Build history of the part. All positions in model axes, mm. A direction names the side the tool comes from. Round coordinates to 2 decimals unless told otherwise and drop trailing zeros. Write each loop counter-clockwise with the first axis right and the second up, starting at its lowest first coordinate (ties: lowest second). Pieces come first, ordered by that corner, then holes. Notation, with made-up numbers: M -6.5,-14.75 L 36.5,-14.75 A16 ccw 36.5,12.25 Z; hole C 41.25,49.25 d11. An arc over 180 degrees is marked long. One line per item, written item: value. Start each with the question number.
```python
from build123d import *

# Parameters (mm, degrees)
SKETCH1_W            = 65
SKETCH1_H            = 56
BOSS_EXTRUDE1_DEPTH  = 2
SKETCH2_R            = 1.375
CUT_EXTRUDE1_DEPTH   = 2
FILLET1_R            = 3
FILLET2_R            = 3
FILLET3_R            = 3
FILLET4_R            = 3
SKETCH3_W            = 50
SKETCH3_H            = 5
BOSS_EXTRUDE2_DEPTH  = 9
SKETCH4_W            = 3
SKETCH4_H            = 22
BOSS_EXTRUDE3_DEPTH  = 6
SKETCH5_W            = 14
SKETCH5_H            = 13
BOSS_EXTRUDE4_DEPTH  = 5
SKETCH6_W            = 6
SKETCH6_H            = 12.1
BOSS_EXTRUDE5_DEPTH  = 6
SKETCH7_R            = 2.5
BOSS_EXTRUDE6_DEPTH  = 3
SKETCH8_W            = 3
SKETCH8_H            = 22
BOSS_EXTRUDE7_DEPTH  = 6
SKETCH9_W            = 16
SKETCH9_H            = 11
BOSS_EXTRUDE8_DEPTH  = 6
SKETCH10_W           = 7
SKETCH10_H           = 6
BOSS_EXTRUDE9_DEPTH  = 3
SKETCH11_W           = 17
SKETCH11_H           = 13
BOSS_EXTRUDE10_DEPTH = 2
SKETCH12_W           = 13
SKETCH12_H           = 13
BOSS_EXTRUDE11_DEPTH = 1


with BuildPart() as part:
    # Sketch1 → Boss-Extrude1 (new body)
    with BuildSketch(Plane(origin=(0, 0, 0), x_dir=(1, 0, 0), z_dir=(0, 1, 0))):
        Rectangle(SKETCH1_W, SKETCH1_H)
    extrude(amount=BOSS_EXTRUDE1_DEPTH)

    # Sketch2 → Cut-Extrude1 (cut)
    with BuildSketch(Plane(origin=(0, 2, 0), x_dir=(1, 0, 0), z_dir=(0, 1, 0))):
        with Locations((-29, -24.5)):
            Circle(SKETCH2_R)
        with Locations((-29, 24.5)):
            Circle(SKETCH2_R)
        with Locations((29, -24.5)):
            Circle(SKETCH2_R)
        with Locations((29, 24.5)):
            Circle(SKETCH2_R)
    extrude(amount=-CUT_EXTRUDE1_DEPTH, mode=Mode.SUBTRACT)

    # Fillet1
    fillet1_edges = [part.edges().sort_by_distance(p)[0] for p in [
        (-32.5, 1, 28),
    ]]
    fillet(fillet1_edges, radius=FILLET1_R)

    # Fillet2
    fillet2_edges = [part.edges().sort_by_distance(p)[0] for p in [
        (32.5, 1, 28),
    ]]
    fillet(fillet2_edges, radius=FILLET2_R)

    # Fillet3
    fillet3_edges = [part.edges().sort_by_distance(p)[0] for p in [
        (32.5, 1, -28),
    ]]
    fillet(fillet3_edges, radius=FILLET3_R)

    # Fillet4
    fillet4_edges = [part.edges().sort_by_distance(p)[0] for p in [
        (-32.5, 1, -28),
    ]]
    fillet(fillet4_edges, radius=FILLET4_R)

    # Sketch3 → Boss-Extrude2 (add)
    with BuildSketch(Plane(origin=(0, 2, 0), x_dir=(1, 0, 0), z_dir=(0, 1, 0))):
        with Locations((0, 24.5)):
            Rectangle(SKETCH3_W, SKETCH3_H)
    extrude(amount=BOSS_EXTRUDE2_DEPTH)

    # Sketch4 → Boss-Extrude3 (add)
    with BuildSketch(Plane(origin=(0, 2, 0), x_dir=(1, 0, 0), z_dir=(0, 1, 0))):
        with Locations((-27.111657831, 3.5)):
            Rectangle(SKETCH4_W, SKETCH4_H)
    extrude(amount=BOSS_EXTRUDE3_DEPTH)

    # Sketch5 → Boss-Extrude4 (add)
    with BuildSketch(Plane(origin=(0, 2, 0), x_dir=(1, 0, 0), z_dir=(0, 1, 0))):
        with Locations((28.469915967, 3.5)):
            Rectangle(SKETCH5_W, SKETCH5_H)
    extrude(amount=BOSS_EXTRUDE4_DEPTH)

    # Sketch6 → Boss-Extrude5 (add)
    with BuildSketch(Plane(origin=(0, 2, 0), x_dir=(1, 0, 0), z_dir=(0, 1, 0))):
        with Locations((20.5, -22.05)):
            Rectangle(SKETCH6_W, SKETCH6_H)
    extrude(amount=BOSS_EXTRUDE5_DEPTH)

    # Sketch7 → Boss-Extrude6 (add)
    with BuildSketch(Plane.XY.offset(28.1)):
        with Locations((20.5, 5)):
            Circle(SKETCH7_R)
    extrude(amount=BOSS_EXTRUDE6_DEPTH)

    # Sketch8 → Boss-Extrude7 (add)
    with BuildSketch(Plane(origin=(0, 2, 0), x_dir=(1, 0, 0), z_dir=(0, 1, 0))):
        with Locations((12.5, -16.9)):
            Rectangle(SKETCH8_W, SKETCH8_H)
    extrude(amount=BOSS_EXTRUDE7_DEPTH)

    # Sketch9 → Boss-Extrude8 (add)
    with BuildSketch(Plane(origin=(0, 2, 0), x_dir=(1, 0, 0), z_dir=(0, 1, 0))):
        with Locations((-0.5, -23.5)):
            Rectangle(SKETCH9_W, SKETCH9_H)
    extrude(amount=BOSS_EXTRUDE8_DEPTH)

    # Sketch10 → Boss-Extrude9 (add)
    with BuildSketch(Plane(origin=(0, 2, 0), x_dir=(1, 0, 0), z_dir=(0, 1, 0))):
        with Locations((-21.9, -26)):
            Rectangle(SKETCH10_W, SKETCH10_H)
    extrude(amount=BOSS_EXTRUDE9_DEPTH)

    # Sketch11 → Boss-Extrude10 (add)
    with BuildSketch(Plane.XZ):
        with Locations((-26, -1.5)):
            Rectangle(SKETCH11_W, SKETCH11_H)
    extrude(amount=BOSS_EXTRUDE10_DEPTH)

    # Sketch12 → Boss-Extrude11 (add)
    with BuildSketch(Plane(origin=(0, 2, 0), x_dir=(1, 0, 0), z_dir=(0, 1, 0))):
        with Locations((-3, 0.5)):
            Rectangle(SKETCH12_W, SKETCH12_H)
    extrude(amount=BOSS_EXTRUDE11_DEPTH)


solid = part.part
```
Item 1: Cut at B-B, the plane z = -13. Write the cut outline in (x, y), plus the area to 3 significant figures.
Item 2: Two-plate mould, pull along X, no slides. Class faces 5 (the flat face through (-3, 3, -1)), 6 (the flat face through (0, 6, -22)), 7 (the flat face through (23.5, 5, 22)): pulls with the +X half, pulls with the -X half, needs draft (parallel to the pull), parting line crosses it, or undercut.
Item 3: Drop flat-ended pins along their axis: pin 1 (17 mm diameter, centred on x = 14, z = -7.5, fed in from -Y); pin 2 (1 mm diameter, centred on y = 1, z = -3, fed in from +X); pin 3 (2.5 mm diameter, centred on x = -21, y = 3.5, fed in from +Z); pin 4 (12 mm diameter, centred on x = -16, z = -17, fed in from +Y). Give the stop position or say it passes through.
Item 4: Cut at A-A, the plane x = 2.5. Write the cut outline in (y, z).
Item 5: Which spindle directions (+Z, -Z, +X, -X, +Y, -Y) get a long thin tool onto all of the face, cutting with end or side? Do faces 1 (the flat face through (-25.4, 3, 26)), 2 (the flat face through (20, 8, 22)), 3 (the flat face through (14, 5, 17)), 4 (the flat face through (28, 4, -10)). Say none if no direction does.
Item 6: Drill centre lines: line 1 (X direction, y = 1.3, z = 24.5) (3 decimals); line 2 (Z direction, x = -29, y = 0.55) (3 decimals); line 3 (Z direction, x = -4, y = 5.75). Where is each one in solid material? Low to high.
Item 7: Cut at D-D, the plane x = -24. Write the cut outline in (y, z).
Item 8: Cut at C-C, the plane y = 4. Count the separate pieces of the cut face and the enclosed holes in it, plus the area to 3 significant figures.
Computed values:
1. outline: M -32.5,0 L 32.5,0 L 32.5,2 L -25.61,2 L -25.61,8 L -28.61,8 L -28.61,2 L -32.5,2 Z
1. area: 148 mm2
2. face 5: undercut
2. face 6: needs draft
2. face 7: pulls with the +X half
3. pin 1: stops at y = 0
3. pin 2: stops at x = 32.5
3. pin 3: stops at z = 29
3. pin 4: stops at y = 11
4. outline: M 0,-28 L 2,-28 L 2,-27 L 11,-27 L 11,-22 L 2,-22 L 2,-7 L 3,-7 L 3,6 L 2,6 L 2,18 L 8,18 L 8,29 L 2,29 L 2,28 L 0,28 Z
5. face 1: +Z, -Z, -X, +Y
5. face 2: +Z, +X, -X, +Y
5. face 3: +Z, +Y
5. face 4: +X, +Y
6. line 1: x = -32.5 to -30.375, -27.625 to 27.625, 30.375 to 32.5
6. line 2: z = -28 to -25.875, -23.125 to 23.125, 25.875 to 28
6. line 3: z = -27 to -22, 18 to 29
7. outline: M -2,-8 L 0,-8 L 0,-28 L 2,-28 L 2,-27 L 11,-27 L 11,-22 L 2,-22 L 2,23 L 5,23 L 5,29 L 2,29 L 2,28 L 0,28 L 0,5 L -2,5 Z
8. separate pieces: 7
8. enclosed holes: 0
8. area: 868 mm2
